```python
from build123d import *

# Parameters (mm, degrees)
SKETCH3_W                = 25.4
SKETCH3_H                = 25.4
BOSS_EXTRUDE1_DEPTH      = 203.2
BOSS_EXTRUDE1_DEPTH_BACK = 203.2
SKETCH4_R                = 2.6035
CUT_EXTRUDE1_DEPTH       = 407.4
CUT_EXTRUDE2_DEPTH       = 407.4
FILLET1_R                = 2.54
FILLET2_R                = 1.778


with BuildPart() as part:
    # Sketch3 → Boss-Extrude1 (new body, two sides)
    with BuildSketch(Plane.XY) as boss_extrude1_sk:
        Rectangle(SKETCH3_W, SKETCH3_H)
    extrude(amount=BOSS_EXTRUDE1_DEPTH)
    extrude(boss_extrude1_sk.sketch, amount=-BOSS_EXTRUDE1_DEPTH_BACK)

    # Sketch4 → Cut-Extrude1 (cut, through all)
    with BuildSketch(Plane.XY.offset(203.2)):
        with BuildLine():
            Line((3.2512, 12.7), (-3.2512, 12.7))
            Line((-3.2512, 12.7), (-3.2512, 10.4902))
            Line((-3.2512, 10.4902), (-6.348478019, 10.4902))
            ThreePointArc((-6.348478019, 10.4902), (-7.335478831, 9.830707141), (-7.103895736, 8.666460301))
            Line((-7.103895736, 8.666460301), (-2.958635435, 4.5212))
            Line((-2.958635435, 4.5212), (2.958635435, 4.5212))
            Line((2.958635435, 4.5212), (7.103895736, 8.666460301))
            ThreePointArc((7.103895736, 8.666460301), (7.335478831, 9.830707141), (6.348478019, 10.4902))
            Line((6.348478019, 10.4902), (3.2512, 10.4902))
            Line((3.2512, 10.4902), (3.2512, 12.7))
        make_face()
        with BuildLine():
            Line((12.7, -3.2512), (12.7, 3.2512))
            Line((12.7, 3.2512), (10.4902, 3.2512))
            Line((10.4902, 3.2512), (10.4902, 6.348478019))
            ThreePointArc((10.4902, 6.348478019), (9.830707141, 7.335478831), (8.666460301, 7.103895736))
            Line((8.666460301, 7.103895736), (4.5212, 2.958635435))
            Line((4.5212, 2.958635435), (4.5212, -2.958635435))
            Line((4.5212, -2.958635435), (8.666460301, -7.103895736))
            ThreePointArc((8.666460301, -7.103895736), (9.830707141, -7.335478831), (10.4902, -6.348478019))
            Line((10.4902, -6.348478019), (10.4902, -3.2512))
            Line((10.4902, -3.2512), (12.7, -3.2512))
        make_face()
        with BuildLine():
            Line((-3.2512, -10.4902), (-3.2512, -12.7))
            Line((-3.2512, -12.7), (3.2512, -12.7))
            Line((3.2512, -12.7), (3.2512, -10.4902))
            Line((3.2512, -10.4902), (6.348478019, -10.4902))
            ThreePointArc((6.348478019, -10.4902), (7.335478831, -9.830707141), (7.103895736, -8.666460301))
            Line((7.103895736, -8.666460301), (2.958635435, -4.5212))
            Line((2.958635435, -4.5212), (-2.958635435, -4.5212))
            Line((-2.958635435, -4.5212), (-7.103895736, -8.666460301))
            ThreePointArc((-7.103895736, -8.666460301), (-7.335478831, -9.830707141), (-6.348478019, -10.4902))
            Line((-6.348478019, -10.4902), (-3.2512, -10.4902))
        make_face()
        with BuildLine():
            Line((-10.4902, 3.2512), (-12.7, 3.2512))
            Line((-12.7, 3.2512), (-12.7, -3.2512))
            Line((-12.7, -3.2512), (-10.4902, -3.2512))
            Line((-10.4902, -3.2512), (-10.4902, -6.348478019))
            ThreePointArc((-10.4902, -6.348478019), (-9.830707141, -7.335478831), (-8.666460301, -7.103895736))
            Line((-8.666460301, -7.103895736), (-4.5212, -2.958635435))
            Line((-4.5212, -2.958635435), (-4.5212, 2.958635435))
            Line((-4.5212, 2.958635435), (-8.666460301, 7.103895736))
            ThreePointArc((-8.666460301, 7.103895736), (-9.830707141, 7.335478831), (-10.4902, 6.348478019))
            Line((-10.4902, 6.348478019), (-10.4902, 3.2512))
        make_face()
        Circle(SKETCH4_R)
    extrude(amount=-CUT_EXTRUDE1_DEPTH, mode=Mode.SUBTRACT)

    # Sketch5 → Cut-Extrude2 (cut, through all)
    with BuildSketch(Plane.XY.offset(203.2)):
        with BuildLine():
            ThreePointArc((-11.5951, 3.2512), (-12.376382283, 3.574817717), (-12.7, 4.3561))
            Line((-12.7, 4.3561), (-12.7, 3.2512))
            Line((-12.7, 3.2512), (-11.5951, 3.2512))
        make_face()
        with BuildLine():
            ThreePointArc((-10.4902, 4.3561), (-10.813817717, 3.574817717), (-11.5951, 3.2512))
            Line((-11.5951, 3.2512), (-10.4902, 3.2512))
            Line((-10.4902, 3.2512), (-10.4902, 4.3561))
        make_face()
        with BuildLine():
            Line((-12.7, -3.2512), (-12.7, -4.3561))
            ThreePointArc((-12.7, -4.3561), (-12.376382283, -3.574817717), (-11.5951, -3.2512))
            Line((-11.5951, -3.2512), (-12.7, -3.2512))
        make_face()
        with BuildLine():
            Line((-10.4902, -3.2512), (-11.5951, -3.2512))
            ThreePointArc((-11.5951, -3.2512), (-10.813817717, -3.574817717), (-10.4902, -4.3561))
            Line((-10.4902, -4.3561), (-10.4902, -3.2512))
        make_face()
        with BuildLine():
            Line((-3.2512, -11.595100007), (-3.2512, -10.4902))
            Line((-3.2512, -10.4902), (-4.3561, -10.4902))
            ThreePointArc((-4.3561, -10.4902), (-3.574817715, -10.81381772), (-3.2512, -11.595100007))
        make_face()
        with BuildLine():
            Line((-3.2512, -12.7), (-3.2512, -11.595100007))
            ThreePointArc((-3.2512, -11.595100007), (-3.57481772, -12.376382285), (-4.3561, -12.7))
            Line((-4.3561, -12.7), (-3.2512, -12.7))
        make_face()
        with BuildLine():
            Line((3.2512, -10.4902), (3.2512, -11.5951))
            ThreePointArc((3.2512, -11.5951), (3.574817718, -10.813817717), (4.3561, -10.4902))
            Line((4.3561, -10.4902), (3.2512, -10.4902))
        make_face()
        with BuildLine():
            Line((3.2512, -12.7), (4.3561, -12.7))
            ThreePointArc((4.3561, -12.7), (3.574817717, -12.376382282), (3.2512, -11.5951))
            Line((3.2512, -11.5951), (3.2512, -12.7))
        make_face()
        with BuildLine():
            Line((11.5951, -3.2512), (10.4902, -3.2512))
            Line((10.4902, -3.2512), (10.4902, -4.3561))
            ThreePointArc((10.4902, -4.3561), (10.813817717, -3.574817717), (11.5951, -3.2512))
        make_face()
        with BuildLine():
            Line((12.7, -3.2512), (11.5951, -3.2512))
            ThreePointArc((11.5951, -3.2512), (12.376382283, -3.574817717), (12.7, -4.3561))
            Line((12.7, -4.3561), (12.7, -3.2512))
        make_face()
        with BuildLine():
            Line((10.4902, 3.2512), (11.5951, 3.2512))
            ThreePointArc((11.5951, 3.2512), (10.813817717, 3.574817717), (10.4902, 4.3561))
            Line((10.4902, 4.3561), (10.4902, 3.2512))
        make_face()
        with BuildLine():
            Line((12.7, 3.2512), (12.7, 4.3561))
            ThreePointArc((12.7, 4.3561), (12.376382283, 3.574817717), (11.5951, 3.2512))
            Line((11.5951, 3.2512), (12.7, 3.2512))
        make_face()
        with BuildLine():
            Line((3.2512, 12.7), (3.2512, 11.595099996))
            ThreePointArc((3.2512, 11.595099996), (3.574817716, 12.376382281), (4.3561, 12.7))
            Line((4.3561, 12.7), (3.2512, 12.7))
        make_face()
        with BuildLine():
            Line((3.2512, 11.595099996), (3.2512, 10.4902))
            Line((3.2512, 10.4902), (4.3561, 10.4902))
            ThreePointArc((4.3561, 10.4902), (3.574817719, 10.813817716), (3.2512, 11.595099996))
        make_face()
        with BuildLine():
            Line((-3.2512, 12.7), (-4.3561, 12.7))
            ThreePointArc((-4.3561, 12.7), (-3.574817717, 12.376382283), (-3.2512, 11.5951))
            Line((-3.2512, 11.5951), (-3.2512, 12.7))
        make_face()
        with BuildLine():
            Line((-3.2512, 10.4902), (-3.2512, 11.5951))
            ThreePointArc((-3.2512, 11.5951), (-3.574817717, 10.813817717), (-4.3561, 10.4902))
            Line((-4.3561, 10.4902), (-3.2512, 10.4902))
        make_face()
        with BuildLine():
            ThreePointArc((-12.7, 5.23875), (-12.14755, 5.7912), (-12.7, 6.34365))
            Line((-12.7, 6.34365), (-12.7, 5.23875))
        make_face()
        with BuildLine():
            ThreePointArc((-12.7, 9.60755), (-12.14755, 10.16), (-12.7, 10.71245))
            Line((-12.7, 10.71245), (-12.7, 9.60755))
        make_face()
        with BuildLine():
            ThreePointArc((-10.71245, 12.7), (-10.16, 12.14755), (-9.60755, 12.7))
            Line((-9.60755, 12.7), (-10.71245, 12.7))
        make_face()
        with BuildLine():
            ThreePointArc((-6.34365, 12.7), (-5.7912, 12.14755), (-5.23875, 12.7))
            Line((-5.23875, 12.7), (-6.34365, 12.7))
        make_face()
        with BuildLine():
            Line((6.34365, 12.7), (5.23875, 12.7))
            ThreePointArc((5.23875, 12.7), (5.7912, 12.14755), (6.34365, 12.7))
        make_face()
        with BuildLine():
            Line((10.71245, 12.7), (9.60755, 12.7))
            ThreePointArc((9.60755, 12.7), (10.16, 12.14755), (10.71245, 12.7))
        make_face()
        with BuildLine():
            Line((12.7, 10.71245), (12.7, 9.60755))
            ThreePointArc((12.7, 9.60755), (12.14755, 10.16), (12.7, 10.71245))
        make_face()
        with BuildLine():
            Line((12.7, 6.34365), (12.7, 5.23875))
            ThreePointArc((12.7, 5.23875), (12.14755, 5.7912), (12.7, 6.34365))
        make_face()
        with BuildLine():
            Line((-12.7, -6.34365), (-12.7, -5.23875))
            ThreePointArc((-12.7, -5.23875), (-12.14755, -5.7912), (-12.7, -6.34365))
        make_face()
        with BuildLine():
            Line((-12.7, -10.71245), (-12.7, -9.60755))
            ThreePointArc((-12.7, -9.60755), (-12.14755, -10.16), (-12.7, -10.71245))
        make_face()
        with BuildLine():
            Line((-10.71245, -12.7), (-9.60755, -12.7))
            ThreePointArc((-9.60755, -12.7), (-10.16, -12.14755), (-10.71245, -12.7))
        make_face()
        with BuildLine():
            Line((-6.34365, -12.7), (-5.23875, -12.7))
            ThreePointArc((-5.23875, -12.7), (-5.7912, -12.14755), (-6.34365, -12.7))
        make_face()
        with BuildLine():
            Line((12.7, -10.71245), (12.7, -9.60755))
            ThreePointArc((12.7, -9.60755), (12.14755, -10.16), (12.7, -10.71245))
        make_face()
        with BuildLine():
            Line((12.7, -6.34365), (12.7, -5.23875))
            ThreePointArc((12.7, -5.23875), (12.14755, -5.7912), (12.7, -6.34365))
        make_face()
        with BuildLine():
            Line((10.71245, -12.7), (9.60755, -12.7))
            ThreePointArc((9.60755, -12.7), (10.16, -12.14755), (10.71245, -12.7))
        make_face()
        with BuildLine():
            Line((6.34365, -12.7), (5.23875, -12.7))
            ThreePointArc((5.23875, -12.7), (5.7912, -12.14755), (6.34365, -12.7))
        make_face()
    extrude(amount=-CUT_EXTRUDE2_DEPTH, mode=Mode.SUBTRACT)

    # Fillet1
    fillet1_edges = [part.edges().sort_by_distance(p)[0] for p in [
        (2.958635435, 4.5212, 0),
        (-2.958635435, 4.5212, 0),
        (-2.958635435, -4.5212, 0),
        (2.958635435, -4.5212, 0),
        (4.5212, -2.958635435, 0),
        (4.5212, 2.958635435, 0),
        (-4.5212, 2.958635435, 0),
        (-4.5212, -2.958635435, 0),
    ]]
    fillet(fillet1_edges, radius=FILLET1_R)

    # Fillet2
    fillet2_edges = [part.edges().sort_by_distance(p)[0] for p in [
        (-12.7, 12.7, 0),
        (12.7, 12.7, 0),
        (12.7, -12.7, 0),
        (-12.7, -12.7, 0),
    ]]
    fillet(fillet2_edges, radius=FILLET2_R)


solid = part.part
```
Can you work these out from the model? Positions are in its coordinate system, mm. Coordinates: 2 decimals unless noted, no trailing zeros. Put each result on its own line as item: value. Start each with the question number.
Q1. I'm going to push flat-ended pins straight in: P1, Ø10, axis at x = 5.5, y = 10, coming from the -Z side; P2, Ø2, axis at y = -1, z = -8, coming from the +X side; P3, Ø3, axis at x = -0.5, z = 42.5, coming from the +Y side; P4, Ø2, axis at x = 1.5, z = 134.5, coming from the -Y side. Where does each tip first touch, or does it pass through?
Q2. Thinking about a two-plate mould opening in Z: for faces 1 (the face through (0, 3, -203.2)), 2 (the face through (0, 3, 203.2)), which applies, pulls with the +Z half, pulls with the -Z half, needs draft (parallel to the pull), parting line crosses it, or undercut?
Q3. If I drill on line 1 (Y direction, x = 0, z = -17.5); line 2 (X direction, y = 0.5, z = -145); line 3 (Y direction, x = -4.25, z = -169), over which ranges is the centre line in solid material (lowest first)? Write a range as [from, to].
Taken from the geometry:
1. P1: stops at z = -203.2
1. P2: stops at x = 4.52
1. P3: stops at y = 4.52
1. P4: stops at y = -4.59
2. face 1: pulls with the -Z half
2. face 2: pulls with the +Z half
3. line 1: y = [-4.52, -2.6], [2.6, 4.52]
3. line 2: x = [-4.52, -2.56], [2.56, 4.52]
3. line 3: y = [-12.69, -10.5], [-5.81, 5.81], [10.5, 12.69]
